from build123d import *

# Parameters (mm, degrees)
SKETCH1_W           = 27
SKETCH1_H           = 44
BOSS_EXTRUDE1_DEPTH = 6
CUT_EXTRUDE1_DEPTH  = 27.5
BOSS_EXTRUDE2_DEPTH = 44
SKETCH4_R           = 2
CUT_EXTRUDE2_DEPTH  = 46.937457483
SKETCH7_R           = 2.05
CUT_EXTRUDE4_DEPTH  = 54.81893677
CUT_EXTRUDE6_DEPTH  = 52.546096044
FILLET1_R           = 1
FILLET2_R           = 3


with BuildPart() as part:
    # Sketch1 → Boss-Extrude1 (new body)
    with BuildSketch(Plane(origin=(0, 0, 0), x_dir=(1, 0, 0), z_dir=(0, 1, 0))):
        Rectangle(SKETCH1_W, SKETCH1_H)
    extrude(amount=BOSS_EXTRUDE1_DEPTH)

    # Sketch2 → Cut-Extrude1 (cut, through all)
    with BuildSketch(Plane(origin=(0, 6, 0), x_dir=(1, 0, 0), z_dir=(0, 1, 0))):
        Polygon((13.5, 22), (-13.5, 6.411542732), (-13.5, 22), align=None)
    extrude(amount=-CUT_EXTRUDE1_DEPTH, mode=Mode.SUBTRACT)

    # Sketch3 → Boss-Extrude2 (add)
    with BuildSketch(Plane(origin=(0, 6, 0), x_dir=(1, 0, 0), z_dir=(0, 1, 0))):
        Polygon((-13.5, 6.411542732), (13.5, 22), (13.5, 16), (-13.5, 0.411542732), align=None)
    extrude(amount=-BOSS_EXTRUDE2_DEPTH)

    # Sketch4 → Cut-Extrude2 (cut, through all)
    with BuildSketch(Plane.XZ):
        with Locations(Location((-4.5, 12, 0), (0, 0, 270))):
            Circle(SKETCH4_R)
        with Locations(Location((5.5, 2, 0), (0, 0, 270))):
            Circle(SKETCH4_R)
    extrude(amount=-CUT_EXTRUDE2_DEPTH, mode=Mode.SUBTRACT)

    # Sketch7 → Cut-Extrude4 (cut, through all)
    with BuildSketch(Plane(origin=(-6.151279442, 0, -10.654328524), x_dir=(-0.8660254037844417, 0, 0.49999999999999495), z_dir=(-0.49999999999999495, 0, -0.8660254037844417))):
        with Locations((-5.514428415, -13)):
            Circle(SKETCH7_R)
        with Locations((-0.514428415, -25.5)):
            Circle(SKETCH7_R)
    extrude(amount=-CUT_EXTRUDE4_DEPTH, mode=Mode.SUBTRACT)

    # Sketch15 → Loft5 section 0
    with BuildSketch(Plane(origin=(9.5, 0, 0), x_dir=(0, 0, -1), z_dir=(1, 0, 0))):
        with BuildLine():
            Line((-22, 0), (13.690598923, 0))
            Line((13.690598923, 0), (13.690598923, -38))
            Line((13.690598923, -38), (-22, -38))
            Line((-22, -38), (-22, 0))
        make_face()
    # Sketch17 → Loft5 section 1
    with BuildSketch(Plane(origin=(13.5, 0, 0), x_dir=(0, 0, -1), z_dir=(1, 0, 0))):
        with BuildLine():
            Line((-22, 0), (16, 0))
            Line((16, 0), (16, -38))
            Line((16, -38), (-22, -38))
            Line((-22, -38), (-22, 0))
        make_face()
    loft()

    # Sketch12 → Loft7 section 0
    with BuildSketch(Plane.ZY.offset(9.5)):
        with BuildLine():
            Line((-2.720943809, -38), (-2.720943809, 0))
            Line((-2.720943809, 0), (22, 0))
            Line((22, 0), (22, -38))
            Line((22, -38), (-2.720943809, -38))
        make_face()
    # Sketch20 → Loft7 section 1
    with BuildSketch(Plane.ZY.offset(13.5)):
        with BuildLine():
            Line((-0.411542732, 0), (22, 0))
            Line((22, 0), (22, -38))
            Line((22, -38), (-0.411542732, -38))
            Line((-0.411542732, -38), (-0.411542732, 0))
        make_face()
    loft()

    # Sketch22 → Cut-Extrude6 (cut, through all)
    with BuildSketch(Plane.ZY.offset(13.5)):
        Polygon((22, 6), (-2.721542732, -38), (22, -38), align=None)
    extrude(amount=-CUT_EXTRUDE6_DEPTH, mode=Mode.SUBTRACT)

    # Fillet1
    fillet1_edges = [part.edges().sort_by_distance(p)[0] for p in [
        (9.5, -19, -13.690598923),
        (-9.5, -18.999467011, -2.720943809),
    ]]
    fillet(fillet1_edges, radius=FILLET1_R)

    # Fillet2
    fillet2_edges = [part.edges().sort_by_distance(p)[0] for p in [
        (-11.408036374, -38, -2.721542732),
        (11.5, -38, -2.721542732),
    ]]
    fillet(fillet2_edges, radius=FILLET2_R)


solid = part.part
The listing builds one solid part. Answer for the finished solid, in the listing's coordinates (mm). A direction names the side the tool comes from. Round coordinates to 2 decimals unless told otherwise and drop trailing zeros. Loops run counter-clockwise (first coordinate to the right, second up) from the corner with the lowest first, then second, coordinate; pieces in that order, holes last. Notation, with made-up numbers: M 21,-39.75 L 33,-39.75 A15 cw 33,-18.75 Z; hole C -21,37 d4. An arc over 180 degrees is marked long. Write each question's results on one line, items separated by ' | '. Start each with the question number.
1) Find section A-A on z = 2.5. Write down the section's boundary in (x, y).
2) Each of these flat-tipped pins is pushed along its axis until it touches: pin 1 (5 mm diameter, centred on x = 10.5, y = -2.5, fed in from -Z); pin 2 (1.5 mm diameter, centred on x = 1.5, y = -3, fed in from -Z). Where does it stop, or does it pass through?
3) Find section C-C on y = -10. Write down the section's boundary in (x, z), plus the area to 3 significant figures.
4) Find section B-B on x = 5.5. Write down the section's boundary in (y, z).
5) Find section D-D on x = -11.25. Write down the section's boundary in (y, z).
6) Straight lines are drawn through the part: probe 1 along X at (y, z) = (-7.5, 7.5); probe 2 along X at (y, z) = (4, 2); probe 3 along Y at (x, z) = (2, 16.5). For each, find the intervals that lie inside material, in ascending order.
7) Determine the mould class of faces 1 (the flat face through (-0.381, -18.734, -7.986)), 2 (the cylindrical face through (-3.12, -24.11, -9.45)), 3 (the flat face through (0, 6, 5)), 4 (the cylindrical face through (0.3, -15, -11.4)) for opening direction Y: pulls with the +Y half, pulls with the -Y half, needs draft (parallel to the pull), parting line crosses it, or undercut.
8) Which of the six approach directions +Z, -Z, +X, -X, +Y, -Y give full straight-line access (tool end or side, diameter ignored) to faces 5 (the flat face through (-9.5, -11, 5)), 6 (the flat face through (13.5, -13, -3))?
Final values:
1) outline: M -13.5,-28.71 L -9.5,-28.71 L -9.5,0 L 3.56,0 L 3.56,6 L -13.5,6 Z; M 7.44,0 L 9.5,0 L 9.5,-28.71 L 13.5,-28.71 L 13.5,6 L 7.44,6 Z
2) pin 1: z = -21.71 | pin 2: z = -15.5
3) outline: M -13.5,-6.41 L 13.5,-22 L 13.5,13.01 L 9.5,13.01 L 9.5,-11.96 A1 cw 8,-12.82 L -9,-3.01 A1 cw -9.5,-2.14 L -9.5,13.01 L -13.5,13.01 Z | area: 332 mm²
4) outline: M -38,-17.38 L 6,-17.38 L 6,0 L 0,0 L 0,-11.38 L -38,-11.38 Z; M 0,4 L 6,4 L 6,22 L 0,18.63 Z
5) outline: M -38,-7.71 L 6,-7.71 L 6,22 L -36.47,-1.86 A3 ccw -38,-4.48 Z
6) probe 1: -13.5 to -9.5, 9.5 to 13.5 | probe 2: -13.5 to 3.5, 7.5 to 13.5 | probe 3: 0 to 6
7) face 1: needs draft | face 2: undercut | face 3: pulls with the +Y half | face 4: undercut
8) face 5: +Z, -Y | face 6: +Z, -Z, +X, +Y, -Y
